Here's the drawing with two shaded views (mm, measured from the low corner). I have some questions. Give positions to 0.01 mm unless a question says otherwise; leave off trailing zeros. Write each loop counter-clockwise with the first axis right and the second up, starting at its lowest first coordinate (ties: lowest second). Pieces come first, ordered by that corner, then holes. Notation, with made-up numbers: (4.5, -18.75) - (20.5, -18.75) arc R28 ccw to (20.5, 7.25) - close; hole circle Ø7 at (75, -17.75). An arc over 180 degrees is marked (long way). Write item = value, one per line.
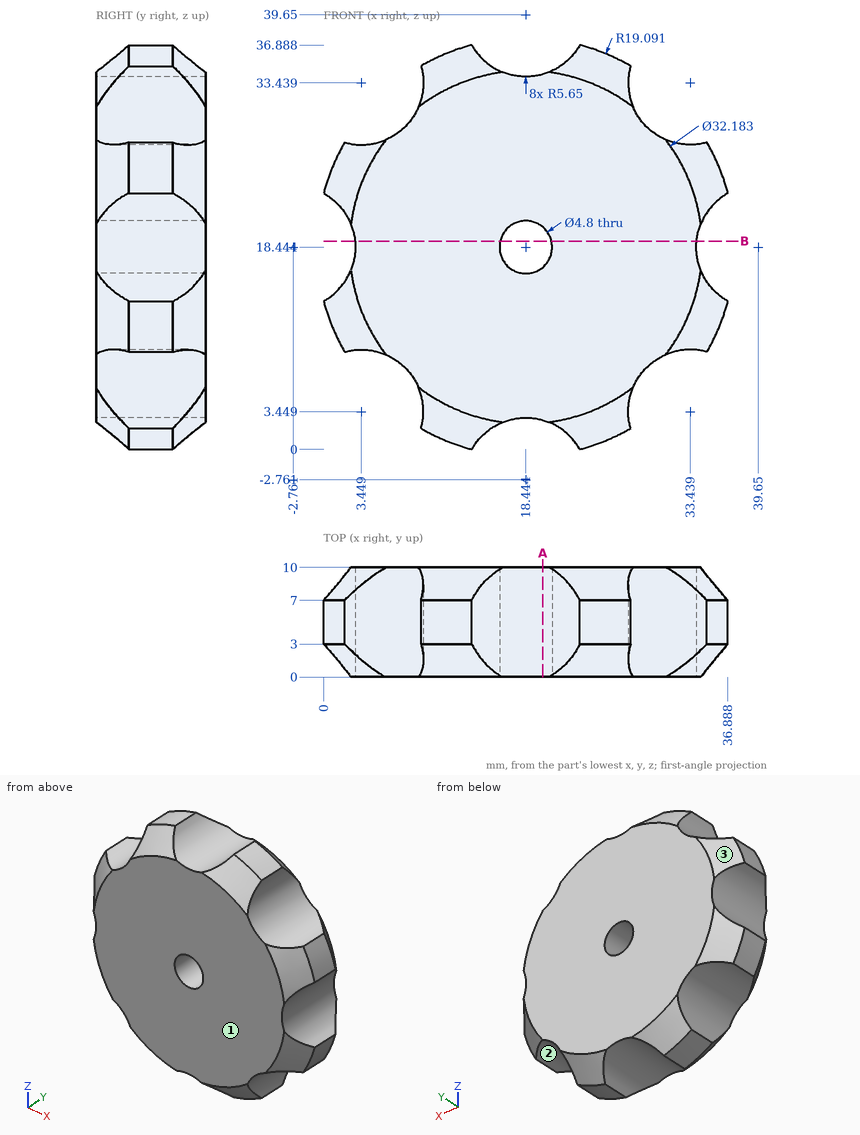
1. Thinking about a two-plate mould opening in X: for the marked faces 1, 2 and 3, which applies, pulls with the +X half, pulls with the -X half, needs draft (parallel to the pull), parting line crosses it, or undercut?
Filled sheet:
face_1 = needs draft
face_2 = undercut
face_3 = pulls with the -X half
2. For pin 1 (2 mm diameter, centred on y = 7, z = 12, fed in from +X); pin 2 (1.5 mm diameter, centred on x = 15, y = 3.5, fed in from +Z) (1 decimal); pin 3 (3 mm diameter, centred on x = 30.5, y = 2.5, fed in from -Z) (1 decimal), each with a flat end and sliding along its axis, tell me the tip position at first contact or that it passes through.
Filled sheet:
pin_1 = 36.74
pin_2 = 35.9
pin_3 = 6.9
3. I need wall thicknesses on line 1 (Z direction, x = 18.5, y = 7.25) (1 decimal); line 2 (Z direction, x = 17.5, y = 8.5); line 3 (X direction, y = 3.5, z = 33.5). Which ranges of each line are inside material? Lowest first, please.
Filled sheet:
line_1 = 2.9 to 16, 20.8 to 34
line_2 = 2.81 to 16.24, 20.65 to 34.08
line_3 = 9.1 to 27.79
4. If we section it at B-B, the plane z = 19: Please give me the cut outline in (x, y).
Filled sheet:
outline = (2.86, 0) - (16.11, 0) - (16.11, 10) - (2.86, 10) - close; (20.78, 0) - (34.03, 0) - (34.03, 10) - (20.78, 10) - close
5. If we section it at A-A, the plane x = 20: Please give me the cut outline in (y, z), and give its area (3 significant figures).
Filled sheet:
outline = (0, 2.67) - (10, 2.67) - (10, 16.62) - (0, 16.62) - close; (0, 20.27) - (10, 20.27) - (10, 34.22) - (0, 34.22) - close
area = 279 mm2
